Geometry check sheet. Reference: drawing and pictorial views, mm from the part's lowest x, y, z. A direction names the side the tool comes from. Round coordinates to 2 decimals unless told otherwise and drop trailing zeros. Write each loop counter-clockwise with the first axis right and the second up, starting at its lowest first coordinate (ties: lowest second). Pieces come first, ordered by that corner, then holes. Notation, with made-up numbers: M 88,44 L 125,44 A31 ccw 125,82 Z; hole C -2,53.25 d9. An arc over 180 degrees is marked long. Use a Markdown table: item, result. Add a question column.
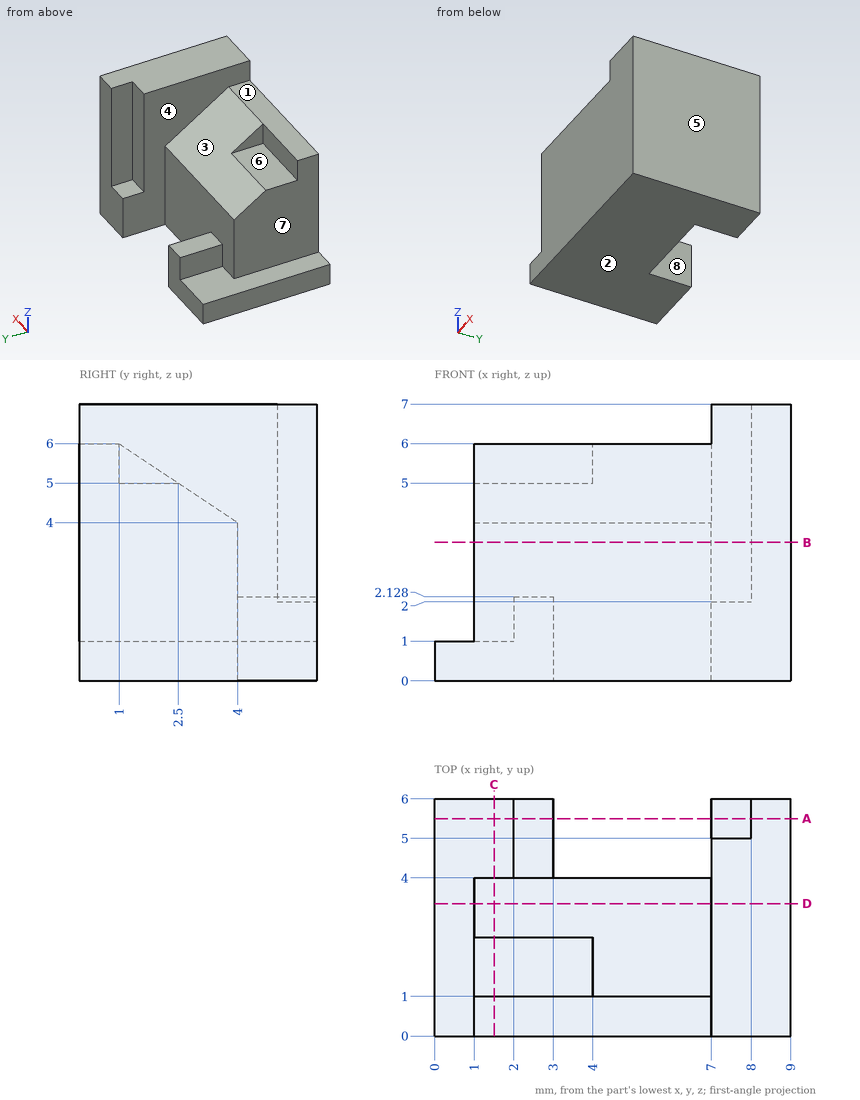
1. Release check for a two-part mould opening along X. For the marked faces 5, 6, 7 and 8 record: +X half, -X half, draft (parallel to the pull), parting line (faces both ways), or undercut.
2. Cross-section at D-D on y = 3.35. Enter the section's corners in (x, z), plus the area to 3 significant figures.
3. Access from +Z, -Z, +X, -X, +Y, -Y to the whole of each face (thin tool, end or side, straight path). Record for the marked faces 1, 2, 3 and 4.
4. Depth check by flat-ended pin: pin 1 Ø3 at (y, z) = (3, 4) entering from -X; pin 2 Ø1 at (x, y) = (1, 4) entering from +Z; pin 3 Ø1.2 at (x, z) = (3, 3) entering from +Y. Enter the tip coordinate at first touch or a pass-through.
5. Cross-section at A-A on y = 5.5. Enter the section's corners in (x, z).
6. Cross-section at B-B on z = 3.5. Enter the section's corners in (x, y).
7. Cross-section at C-C on x = 1.5. Enter the section's corners in (y, z).
8. Scan lines: line 1 along X through (y, z) = (4.5, 0.5); line 2 along X through (y, z) = (0.9, 2.5); line 3 along Z through (x, y) = (2.5, 5.35). Record each from-to range of solid material in increasing order. Write a range as from..to.
Answer:
| question | item | result |
|---|---|---|
| 1 | face 5 | +X half |
| 1 | face 6 | draft |
| 1 | face 7 | -X half |
| 1 | face 8 | undercut |
| 2 | outline | M 0,0 L 9,0 L 9,7 L 7,7 L 7,4.43 L 1,4.43 L 1,1 L 0,1 Z |
| 2 | area | 41.6 mm^2 |
| 3 | face 1 | +Z, -X, +Y, -Y |
| 3 | face 2 | -Z, +X, -X, +Y, -Y |
| 3 | face 3 | +Z, -X, +Y |
| 3 | face 4 | +Z, +Y |
| 4 | pin 1 | stops at x = 1 |
| 4 | pin 2 | stops at z = 4.33 |
| 4 | pin 3 | stops at y = 4 |
| 5 | outline | M 0,0 L 3,0 L 3,2.13 L 2,2.13 L 2,1 L 0,1 Z; M 7,0 L 9,0 L 9,7 L 8,7 L 8,2 L 7,2 Z |
| 6 | outline | M 1,0 L 9,0 L 9,6 L 8,6 L 8,5 L 7,5 L 7,4 L 1,4 Z |
| 7 | outline | M 0,0 L 6,0 L 6,1 L 4,1 L 4,4 L 2.5,5 L 1,5 L 1,6 L 0,6 Z |
| 8 | line 1 | x = 0..3, 7..9 |
| 8 | line 2 | x = 1..9 |
| 8 | line 3 | z = 0..2.13 |
